Build history of the part. All positions in model axes, mm. Round coordinates to 2 decimals unless told otherwise and drop trailing zeros. Order: outer loops, then holes, each group sorted by start corner. A loop starts at its lowest first (then second) coordinate and runs counter-clockwise, first axis right, second up. Notation, with made-up numbers: M 27,-22 L 55,-22 A36 cw 55,14 Z; hole C 10,19 d11. An arc over 180 degrees is marked long. One line per item, written item: value. Start each with the question number.
Item 1: Probe L1, parallel to X at y = 21.5, z = 1.75; L2, parallel to Y at x = 4, z = 1.75; L3, parallel to Y at x = 4.5, z = 0.1. List the from-to ranges inside material, lowest first.
Item 2: Band-saw the part on A-A, the plane x = 25.25. Write the cut outline in (y, z).
Item 3: Band-saw the part on C-C, the plane x = 3.78. Write the cut outline in (y, z).
Item 4: Band-saw the part on B-B, the plane z = 0.35. Write the cut outline in (x, y), then the cut area to 3 significant figures.
Item 5: Two-plate mould, pull along X, no slides. Class faces 1 (the flat face through (14, 24.377, 1)), 2 (the cylindrical face through (24.08, -2.95, 0.99)), 3 (the flat face through (28.6, 11, 1)), 4 (the flat face through (0, 10, 1)): +X half, -X half, draft (parallel to the pull), parting line (faces both ways), or undercut.
Item 6: Pin check, flat tip, straight feed: pin 1 (2.5 mm diameter, centred on x = 24.82, y = -3.62, fed in from -Z). Stop position of the tip, or through.
Item 7: Band-saw the part on D-D, the plane x = 20.75. Write the cut outline in (y, z).
```python
from build123d import *

# Parameters (mm, degrees)
SKETCH_1_R      = 1
EXTRUDE_1_DEPTH = 2


with BuildPart() as part:
    # 草图1 → 凸台-拉伸1 (new body)
    with BuildSketch(Plane.XY):
        with BuildLine():
            Line((0, 24.376794113), (28.6, 24.376794113))
            Line((28.6, 24.376794113), (28.6, -3.62321671))
            ThreePointArc((28.6, -3.62321671), (24.411626971, -13.734843681), (14.3, -17.92321671))
            ThreePointArc((14.3, -17.92321671), (4.188373029, -13.734843681), (0, -3.62321671))
            Line((0, -3.62321671), (0, 24.376794113))
        make_face()
        with Locations((24.78, 21.376794113)):
            Circle(SKETCH_1_R, mode=Mode.SUBTRACT)
        with Locations((3.78, 21.376794113)):
            Circle(SKETCH_1_R, mode=Mode.SUBTRACT)
        with Locations((3.82, -3.623205887)):
            Circle(SKETCH_1_R, mode=Mode.SUBTRACT)
        with Locations((24.82, -3.623205887)):
            Circle(SKETCH_1_R, mode=Mode.SUBTRACT)
    extrude(amount=EXTRUDE_1_DEPTH)


solid = part.part
```
Output:
1. L1: x = 0 to 2.79, 4.77 to 23.79, 25.77 to 28.6
1. L2: y = -13.54 to -4.61, -2.64 to 20.4, 22.35 to 24.38
1. L3: y = -14.04 to -4.36, -2.89 to 20.68, 22.07 to 24.38
2. outline: M -12.82,0 L -4.53,0 L -4.53,2 L -12.82,2 Z; M -2.72,0 L 20.49,0 L 20.49,2 L -2.72,2 Z; M 22.26,0 L 24.38,0 L 24.38,2 L 22.26,2 Z
3. outline: M -13.31,0 L -4.62,0 L -4.62,2 L -13.31,2 Z; M -2.62,0 L 20.38,0 L 20.38,2 L -2.62,2 Z; M 22.38,0 L 24.38,0 L 24.38,2 L 22.38,2 Z
4. outline: M 0,-3.62 A14.3 ccw 28.6,-3.62 L 28.6,24.38 L 0,24.38 Z; hole C 3.78,21.38 d2; hole C 3.82,-3.62 d2; hole C 24.78,21.38 d2; hole C 24.82,-3.62 d2
4. area: 1,110 mm²
5. face 1: draft
5. face 2: undercut
5. face 3: +X half
5. face 4: -X half
6. pin 1: stops at z = 0
7. outline: M -16.39,0 L 24.38,0 L 24.38,2 L -16.39,2 Z
